from build123d import *

# Parameters (mm, degrees)
SKETCH1_R           = 3
BOSS_EXTRUDE1_DEPTH = 3.175
FILLET1_R           = 10
FILLET2_R           = 30


with BuildPart() as part:
    # Sketch1 → Boss-Extrude1 (new body)
    with BuildSketch(Plane.XY):
        with BuildLine():
            Line((-95, -40), (-25, -40))
            ThreePointArc((-25, -40), (0, -57.5), (25, -40))
            Line((25, -40), (95, -40))
            Line((95, -40), (95, 40))
            Line((95, 40), (25, 40))
            ThreePointArc((25, 40), (0, 57.5), (-25, 40))
            Line((-25, 40), (-95, 40))
            Line((-95, 40), (-95, -40))
        make_face()
        with Locations((0, 42.5)):
            Circle(SKETCH1_R, mode=Mode.SUBTRACT)
        with Locations((0, -42.5)):
            Circle(SKETCH1_R, mode=Mode.SUBTRACT)
        with BuildLine():
            Line((30, 27.5), (80, 27.5))
            ThreePointArc((80, 27.5), (82.5, 25), (80, 22.5))
            Line((80, 22.5), (30, 22.5))
            ThreePointArc((30, 22.5), (27.5, 25), (30, 27.5))
        make_face(mode=Mode.SUBTRACT)
        with BuildLine():
            Line((30, -27.5), (80, -27.5))
            ThreePointArc((80, -27.5), (82.5, -25), (80, -22.5))
            Line((80, -22.5), (30, -22.5))
            ThreePointArc((30, -22.5), (27.5, -25), (30, -27.5))
        make_face(mode=Mode.SUBTRACT)
        with BuildLine():
            Line((-30, 27.5), (-80, 27.5))
            ThreePointArc((-80, 27.5), (-82.5, 25), (-80, 22.5))
            Line((-80, 22.5), (-30, 22.5))
            ThreePointArc((-30, 22.5), (-27.5, 25), (-30, 27.5))
        make_face(mode=Mode.SUBTRACT)
        with BuildLine():
            Line((-30, -27.5), (-80, -27.5))
            ThreePointArc((-80, -27.5), (-82.5, -25), (-80, -22.5))
            Line((-80, -22.5), (-30, -22.5))
            ThreePointArc((-30, -22.5), (-27.5, -25), (-30, -27.5))
        make_face(mode=Mode.SUBTRACT)
    extrude(amount=BOSS_EXTRUDE1_DEPTH)

    # Fillet1
    fillet1_edges = [part.edges().sort_by_distance(p)[0] for p in [
        (95, 40, 1.5875),
        (95, -40, 1.5875),
        (-95, -40, 1.5875),
        (-95, 40, 1.5875),
    ]]
    fillet(fillet1_edges, radius=FILLET1_R)

    # Fillet2
    fillet2_edges = [part.edges().sort_by_distance(p)[0] for p in [
        (25, -40, 1.5875),
        (-25, -40, 1.5875),
        (-25, 40, 1.5875),
        (25, 40, 1.5875),
    ]]
    fillet(fillet2_edges, radius=FILLET2_R)


solid = part.part
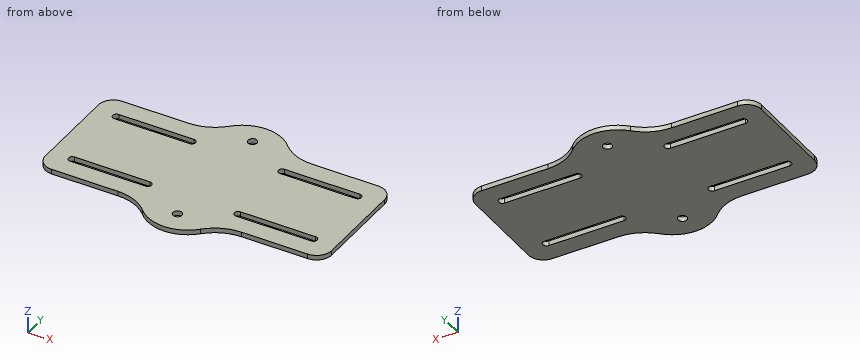
CAD build for the part. Positions are in the model's coordinates, mm. Coordinates: 2 decimals unless noted, no trailing zeros. Write each loop counter-clockwise with the first axis right and the second up, starting at its lowest first coordinate (ties: lowest second). Pieces come first, ordered by that corner, then holes. Notation, with made-up numbers: M -23,28.5 L 34,28.5 A17 cw 34,60.5 Z; hole C 62,-6.5 d5. An arc over 180 degrees is marked long. Return JSON: item names as keys, results as strings.
Item 1: Slice it at D-D, the plane y = -42.5. Write the cut outline in (x, z) (3 decimals).
Findings below:
{"outline": "M -28.937,0 L -3,0 L -3,3.175 L -28.937,3.175 Z; M 3,0 L 28.937,0 L 28.937,3.175 L 3,3.175 Z"}
Item 2: Probe line 1 (Y direction, x = 79, z = 2.8); line 2 (Y direction, x = 33, z = 1.4); line 3 (X direction, y = 45, z = 1.5). List the from-to ranges inside material, lowest first. Write a range as from..to.
Findings below:
{"line 1": "y = -40..-27.5, -22.5..22.5, 27.5..40", "line 2": "y = -41.07..-27.5, -22.5..22.5, 27.5..41.07", "line 3": "x = -24.34..-1.66, 1.66..24.34"}
Item 3: Drop flat-ended pins along their axis: pin 1 Ø1.6 at (x, z) = (58.5, 1) entering from -Y; pin 2 Ø1.6 at (x, z) = (61, 2) entering from +Y. Give the stop position or say it passes through.
Findings below:
{"pin 1": "stops at y = -40", "pin 2": "stops at y = 40"}
Item 4: Slice it at A-A, the plane y = -25. Write the cut outline in (x, z) (3 decimals).
Findings below:
{"outline": "M -95,0 L -82.5,0 L -82.5,3.175 L -95,3.175 Z; M -27.5,0 L 27.5,0 L 27.5,3.175 L -27.5,3.175 Z; M 82.5,0 L 95,0 L 95,3.175 L 82.5,3.175 Z"}
Item 5: Slice it at B-B, the plane z = 2.25. State how many separate pieces and enclosed holes the cut face has, and give its area (3 significant figures).
Findings below:
{"separate pieces": "1", "enclosed holes": "6", "area": "15,400 mm2"}
Item 6: Slice it at C-C, the plane x = 0. Write the cut outline in (y, z) (3 decimals), and give its area (3 significant figures).
Findings below:
{"outline": "M -57.5,0 L -45.5,0 L -45.5,3.175 L -57.5,3.175 Z; M -39.5,0 L 39.5,0 L 39.5,3.175 L -39.5,3.175 Z; M 45.5,0 L 57.5,0 L 57.5,3.175 L 45.5,3.175 Z", "area": "327 mm2"}
